```python
from build123d import *

# Parameters (mm, degrees)
SKETCH2_W           = 75
SKETCH2_H           = 25
BOSS_EXTRUDE1_DEPTH = 3
BOSS_EXTRUDE2_DEPTH = 30
SKETCH4_W           = 6
SKETCH4_H           = 30
BOSS_EXTRUDE3_DEPTH = 6
SKETCH5_W           = 6
SKETCH5_H           = 30
BOSS_EXTRUDE4_DEPTH = 6
SKETCH6_R           = 1.75
CUT_EXTRUDE1_DEPTH  = 16
BOSS_EXTRUDE5_DEPTH = 6
FILLET1_R           = 0.5
FILLET2_R           = 0.5


with BuildPart() as part:
    # Sketch2 → Boss-Extrude1 (new body)
    with BuildSketch(Plane(origin=(0, 0, 0), x_dir=(1, 0, 0), z_dir=(0, 1, 0))):
        with Locations((0, 12.5)):
            Rectangle(SKETCH2_W, SKETCH2_H)
    extrude(amount=BOSS_EXTRUDE1_DEPTH)

    # Sketch3 → Boss-Extrude2 (add)
    with BuildSketch(Plane(origin=(0, 3, 0), x_dir=(1, 0, 0), z_dir=(0, 1, 0))):
        Polygon((-35.5, 25), (-35.5, 2), (35.5, 2), (35.5, 25), (37.5, 25), (37.5, 0), (-37.5, 0), (-37.5, 25), align=None)
    extrude(amount=BOSS_EXTRUDE2_DEPTH)

    # Sketch4 → Boss-Extrude3 (add)
    with BuildSketch(Plane(origin=(37.5, 0, 0), x_dir=(0, 0, -1), z_dir=(1, 0, 0))):
        with Locations((22, 18)):
            Rectangle(SKETCH4_W, SKETCH4_H)
    extrude(amount=BOSS_EXTRUDE3_DEPTH)

    # Sketch5 → Boss-Extrude4 (add)
    with BuildSketch(Plane.ZY.offset(37.5)):
        with Locations((-22, 18)):
            Rectangle(SKETCH5_W, SKETCH5_H)
    extrude(amount=BOSS_EXTRUDE4_DEPTH)

    # Sketch6 → Cut-Extrude1 (cut)
    with BuildSketch(Plane(origin=(0, 0, -25), x_dir=(-1, 0, 0), z_dir=(0, 0, -1))):
        with Locations((-40.5, 29)):
            Circle(SKETCH6_R)
        with Locations((40.5, 29)):
            Circle(SKETCH6_R)
        with Locations((-40.5, 19)):
            Circle(SKETCH6_R)
        with Locations((-40.5, 9)):
            Circle(SKETCH6_R)
        with Locations((40.5, 19)):
            Circle(SKETCH6_R)
        with Locations((40.5, 9)):
            Circle(SKETCH6_R)
    extrude(amount=-CUT_EXTRUDE1_DEPTH, mode=Mode.SUBTRACT)

    # Sketch7 → Boss-Extrude5 (add)
    with BuildSketch(Plane(origin=(0, 0, -25), x_dir=(-1, 0, 0), z_dir=(0, 0, -1))):
        Polygon((35.5, 33), (36.5, 33), (36.5, 2), (-36.5, 2), (-36.5, 33), (-35.5, 33), (-35.5, 3), (35.5, 3), align=None)
    extrude(amount=BOSS_EXTRUDE5_DEPTH)

    # Fillet1
    fillet1_edges = [part.edges().sort_by_distance(p)[0] for p in [
        (35.5, 18, -2),
        (-35.5, 18, -2),
    ]]
    fillet(fillet1_edges, radius=FILLET1_R)

    # Fillet2
    fillet2_edges = [part.edges().sort_by_distance(p)[0] for p in [
        (37.5, 16.5, 0),
        (-37.5, 16.5, 0),
    ]]
    fillet(fillet2_edges, radius=FILLET2_R)


solid = part.part
```
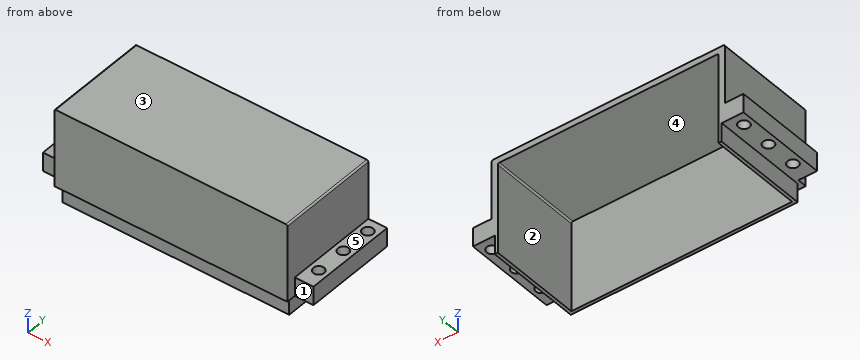
Build history of the part. All positions in model axes, mm. Face numbers are marked on the shaded views. A direction names the side the tool comes from. Coordinates: 2 decimals unless noted, no trailing zeros. Order: outer loops, then holes, each group sorted by start corner. A loop starts at its lowest first (then second) coordinate and runs counter-clockwise, first axis right, second up. Notation, with made-up numbers: (47, 31) -> (98, 31) arc R11 cw to (98, 46) -> close; hole circle Ø6 at (69.25, -20.5). An arc over 180 degrees is marked (long way). Answer in a Markdown table with one row per item. Add a question column.
Q1. Band-saw the part on B-B, the plane y = 29. List the corners of the cut face in (x, z), then the cut area to 3 significant figures.
Q2. Drop flat-ended pins along their axis: pin 1 (4 mm diameter, centred on x = -40.5, y = 29, fed in from +Z); pin 2 (6 mm diameter, centred on y = 18.5, z = -14, fed in from -X); pin 3 (1.8 mm diameter, centred on y = 15, z = -27.5, fed in from -X). Give the stop position or say it passes through.
Q3. Band-saw the part on A-A, the plane x = -40.5. List the corners of the cut face in (y, z).
Q4. Mould opens along X. For the marked faces 4 and 5 say: +X half, -X half, draft (parallel to the pull), parting line (faces both ways), or undercut.
Q5. Wall check: line 1 along Y through (x, z) = (40.5, -21); line 2 along X through (y, z) = (21.5, -5.5); line 3 along Y through (x, z) = (19.5, -19.5). Give the ranges that are in metal, low to high. Write a range as [from, to].
Q6. Which spindle directions (+Z, -Z, +X, -X, +Y, -Y) get a long thin tool onto all of the face, cutting with end or side? Do the marked faces 1, 2 and 3. Say none if no direction does.
Q7. Band-saw the part on C-C, the plane x = -19. List the corners of the cut face in (y, z), then the cut area to 3 significant figures.
Q8. Band-saw the part on D-D, the plane z = -28. List the corners of the cut face in (x, y), then the cut area to 3 significant figures.
Answers follow:
| question | item | result |
|---|---|---|
| 1 | outline | (-43.5, -25) -> (-42.25, -25) -> (-42.25, -19) -> (-43.5, -19) -> close; (-38.75, -25) -> (-36.5, -25) -> (-36.5, -31) -> (-35.5, -31) -> (-35.5, -2.5) arc R0.5 cw to (-35, -2) -> (35, -2) arc R0.5 cw to (35.5, -2.5) -> (35.5, -31) -> (36.5, -31) -> (36.5, -25) -> (38.75, -25) -> (38.75, -19) -> (37.5, -19) -> (37.5, -0.5) arc R0.5 ccw to (37, 0) -> (-37, 0) arc R0.5 ccw to (-37.5, -0.5) -> (-37.5, -19) -> (-38.75, -19) -> close; (42.25, -25) -> (43.5, -25) -> (43.5, -19) -> (42.25, -19) -> close |
| 1 | area | 284 mm^2 |
| 2 | pin 1 | z = -19 |
| 2 | pin 2 | x = -37.5 |
| 2 | pin 3 | x = -36.5 |
| 3 | outline | (3, -25) -> (7.25, -25) -> (7.25, -19) -> (3, -19) -> close; (10.75, -25) -> (17.25, -25) -> (17.25, -19) -> (10.75, -19) -> close; (20.75, -25) -> (27.25, -25) -> (27.25, -19) -> (20.75, -19) -> close; (30.75, -25) -> (33, -25) -> (33, -19) -> (30.75, -19) -> close |
| 4 | face 4 | undercut |
| 4 | face 5 | draft |
| 5 | line 1 | [3, 7.25], [10.75, 17.25], [20.75, 27.25], [30.75, 33] |
| 5 | line 2 | [-37.5, -35.5], [35.5, 37.5] |
| 5 | line 3 | [0, 3] |
| 6 | face 1 | +Z, -Z, +X, -Y |
| 6 | face 2 | -Z, +Y |
| 6 | face 3 | +Z, +X, -X, +Y, -Y |
| 7 | outline | (0, -25) -> (2, -25) -> (2, -31) -> (3, -31) -> (3, -2) -> (33, -2) -> (33, 0) -> (0, 0) -> close |
| 7 | area | 141 mm^2 |
| 8 | outline | (-36.5, 2) -> (36.5, 2) -> (36.5, 33) -> (35.5, 33) -> (35.5, 3) -> (-35.5, 3) -> (-35.5, 33) -> (-36.5, 33) -> close |
| 8 | area | 133 mm^2 |
